from build123d import *

# Parameters (mm, degrees)
F0_R     = 22.5
F0_R_2   = 19
F0_R_3   = 16.25
F0_R_4   = 1
F0_R_5   = 11
F0_R_6   = 10
F0_R_7   = 8
F0_R_8   = 6.4
F0_R_9   = 3.8
F0_R_10  = 2.875
F1_DEPTH = 1.15
F2_DEPTH = 7.65
F3_DEPTH = 3.5
F4_DEPTH = 3.1
F5_DEPTH = 5.4
F6_DEPTH = 8.8
F7_R     = 3.5


with BuildPart() as f1:
    # F0 (on Top) → F1 (new body)
    with BuildSketch(Plane.XY):
        Circle(F0_R)
        Circle(F0_R_2, mode=Mode.SUBTRACT)
        Circle(F0_R_2)
        Circle(F0_R_3, mode=Mode.SUBTRACT)
        Circle(F0_R_3)
        with BuildLine():
            ThreePointArc((8.26016, -11.550314), (0, -14.2), (-8.26016, -11.550314))
            ThreePointArc((-8.26016, -11.550314), (-10.960155, -10.960155), (-11.550314, -8.26016))
            ThreePointArc((-11.550314, -8.26016), (-14.2, 0), (-11.550314, 8.26016))
            ThreePointArc((-11.550314, 8.26016), (-10.960155, 10.960155), (-8.26016, 11.550314))
            ThreePointArc((-8.26016, 11.550314), (0, 14.2), (8.26016, 11.550314))
            ThreePointArc((8.26016, 11.550314), (10.960155, 10.960155), (11.550314, 8.26016))
            ThreePointArc((11.550314, 8.26016), (14.2, 0), (11.550314, -8.26016))
            ThreePointArc((11.550314, -8.26016), (10.960155, -10.960155), (8.26016, -11.550314))
        make_face(mode=Mode.SUBTRACT)
        with BuildLine():
            ThreePointArc((-11.550314, -8.26016), (-10.960155, -10.960155), (-8.26016, -11.550314))
            ThreePointArc((-8.26016, -11.550314), (0, -14.2), (8.26016, -11.550314))
            ThreePointArc((8.26016, -11.550314), (10.960155, -10.960155), (11.550314, -8.26016))
            ThreePointArc((11.550314, -8.26016), (14.2, 0), (11.550314, 8.26016))
            ThreePointArc((11.550314, 8.26016), (10.960155, 10.960155), (8.26016, 11.550314))
            ThreePointArc((8.26016, 11.550314), (0, 14.2), (-8.26016, 11.550314))
            ThreePointArc((-8.26016, 11.550314), (-10.960155, 10.960155), (-11.550314, 8.26016))
            ThreePointArc((-11.550314, 8.26016), (-14.2, 0), (-11.550314, -8.26016))
        make_face()
        with Locations((-9.15, -9.15)):
            Circle(F0_R_4, mode=Mode.SUBTRACT)
        with Locations((9.15, -9.15)):
            Circle(F0_R_4, mode=Mode.SUBTRACT)
        with Locations((-9.15, 9.15)):
            Circle(F0_R_4, mode=Mode.SUBTRACT)
        Circle(F0_R_5, mode=Mode.SUBTRACT)
        with Locations((9.15, 9.15)):
            Circle(F0_R_4, mode=Mode.SUBTRACT)
        Circle(F0_R_5)
        Circle(F0_R_6, mode=Mode.SUBTRACT)
        Circle(F0_R_6)
        Circle(F0_R_7, mode=Mode.SUBTRACT)
        Circle(F0_R_7)
        Circle(F0_R_8, mode=Mode.SUBTRACT)
        with Locations((-9.15, 9.15)):
            Circle(F0_R_4)
        with Locations((9.15, 9.15)):
            Circle(F0_R_4)
        with Locations((9.15, -9.15)):
            Circle(F0_R_4)
        with Locations((-9.15, -9.15)):
            Circle(F0_R_4)
        Circle(F0_R_8)
        Circle(F0_R_9, mode=Mode.SUBTRACT)
        Circle(F0_R_9)
        Circle(F0_R_10, mode=Mode.SUBTRACT)
    extrude(amount=F1_DEPTH)

    # F0 (on Top) → F2 (join)
    with BuildSketch(Plane.XY):
        Circle(F0_R_2)
        Circle(F0_R_3, mode=Mode.SUBTRACT)
    extrude(amount=F2_DEPTH)

    # F0 (on Top) → F3 (join)
    with BuildSketch(Plane.XY):
        with BuildLine():
            ThreePointArc((-11.550314, -8.26016), (-10.960155, -10.960155), (-8.26016, -11.550314))
            ThreePointArc((-8.26016, -11.550314), (0, -14.2), (8.26016, -11.550314))
            ThreePointArc((8.26016, -11.550314), (10.960155, -10.960155), (11.550314, -8.26016))
            ThreePointArc((11.550314, -8.26016), (14.2, 0), (11.550314, 8.26016))
            ThreePointArc((11.550314, 8.26016), (10.960155, 10.960155), (8.26016, 11.550314))
            ThreePointArc((8.26016, 11.550314), (0, 14.2), (-8.26016, 11.550314))
            ThreePointArc((-8.26016, 11.550314), (-10.960155, 10.960155), (-11.550314, 8.26016))
            ThreePointArc((-11.550314, 8.26016), (-14.2, 0), (-11.550314, -8.26016))
        make_face()
        with Locations((-9.15, -9.15)):
            Circle(F0_R_4, mode=Mode.SUBTRACT)
        with Locations((9.15, -9.15)):
            Circle(F0_R_4, mode=Mode.SUBTRACT)
        with Locations((-9.15, 9.15)):
            Circle(F0_R_4, mode=Mode.SUBTRACT)
        Circle(F0_R_5, mode=Mode.SUBTRACT)
        with Locations((9.15, 9.15)):
            Circle(F0_R_4, mode=Mode.SUBTRACT)
        Circle(F0_R_6)
        Circle(F0_R_7, mode=Mode.SUBTRACT)
    extrude(amount=-F3_DEPTH)

    # F0 (on Top) → F4 (join)
    with BuildSketch(Plane.XY):
        Circle(F0_R_5)
        Circle(F0_R_6, mode=Mode.SUBTRACT)
    extrude(amount=-F4_DEPTH)

    # F0 (on Top) → F5 (join)
    with BuildSketch(Plane.XY):
        Circle(F0_R_7)
        Circle(F0_R_8, mode=Mode.SUBTRACT)
        Circle(F0_R_8)
        Circle(F0_R_9, mode=Mode.SUBTRACT)
    extrude(amount=-F5_DEPTH)

    # F0 (on Top) → F6 (join)
    with BuildSketch(Plane.XY):
        Circle(F0_R_9)
        Circle(F0_R_10, mode=Mode.SUBTRACT)
    extrude(amount=-F6_DEPTH)

    # F7
    f7_edges = [f1.edges().sort_by_distance(p)[0] for p in [
        (-2.875, 0, 1.15),
    ]]
    fillet(f7_edges, radius=F7_R)


solid = f1.part
Work out the finished part from the listing and answer in its coordinate system (mm). A direction names the side the tool comes from. Give positions to 0.01 mm unless a question says otherwise; leave off trailing zeros. Loops run counter-clockwise (first coordinate to the right, second up) from the corner with the lowest first, then second, coordinate; pieces in that order, holes last. Notation, with made-up numbers: (32, 61) -> (90, 61) arc R26 ccw to (90, 88) -> close; hole circle Ø8 at (57, 70.25). An arc over 180 degrees is marked (long way). Use a Markdown table: item, result. Add a question column.
1. Flat-ended cylindrical pins translate along their axes: pin 1 Ø2 at (x, z) = (3.5, 5) entering from -Y; pin 2 Ø17.5 at (x, y) = (3, 3) entering from -Z; pin 3 Ø4 at (x, y) = (-6, 13.5) entering from -Z; pin 4 Ø1.5 at (x, y) = (-13, 4) entering from +Z. Find the tip coordinate at first contact, or state that the pin passes through.
2. Section A-A on z = -6 is taken. Determine the outline of the cut face in (x, y) (3 decimals).
3. Section D-D on z = 4.75 is taken. Determine the outline of the cut face in (x, y).
4. Determine the mould class of faces 5 (the flat face through (-9, -9, 0)), 6 (the cylindrical face through (10.382, -19.961, 0.567)), 7 (the flat face through (0, 8.2, -3.5)), 8 (the cylindrical face through (15.5, 4.88, 4.35)) for opening direction Y: released by +Y, released by -Y, zero draft, split by the parting line, or undercut.
5. For faces 1 (the flat face through (7, 0, 1.15)), 2 (the flat face through (-9, 9, 0)), 3 (the cylindrical face through (14.2, -0.1, -1.7)), 4 (the cylindrical face through (2.742, 0.864, -5.53)), determine the directions among +Z, -Z, +X, -X, +Y, -Y from which every point of the face is accessible in a straight line to the end or side of a thin tool.
6. Find the intervals of material crossed by probe 1 along Y at (x, z) = (-9.15, -2.55); probe 2 along Y at (x, z) = (0, -7) (3 decimals); probe 3 along Z at (x, y) = (5, 12), in increasing order.
Results below:
| question | item | result |
|---|---|---|
| 1 | pin 1 | stops at y = -18.83 |
| 1 | pin 2 | stops at z = -8.8 |
| 1 | pin 3 | stops at z = -3.5 |
| 1 | pin 4 | stops at z = 1.15 |
| 2 | outline | circle Ø7.6 at (0, 0); hole circle Ø5.75 at (0, 0) |
| 3 | outline | circle Ø38 at (0, 0); hole circle Ø32.5 at (0, 0) |
| 4 | face 5 | undercut |
| 4 | face 6 | split by the parting line |
| 4 | face 7 | zero draft |
| 4 | face 8 | undercut |
| 5 | face 1 | +Z |
| 5 | face 2 | -Z |
| 5 | face 3 | -Z, +X |
| 5 | face 4 | +Z, -Z |
| 6 | probe 1 | y = -11.71 to -10.15, -8.15 to 8.15, 10.15 to 11.71 |
| 6 | probe 2 | y = -3.8 to -2.875, 2.875 to 3.8 |
| 6 | probe 3 | z = -3.5 to 1.15 |
